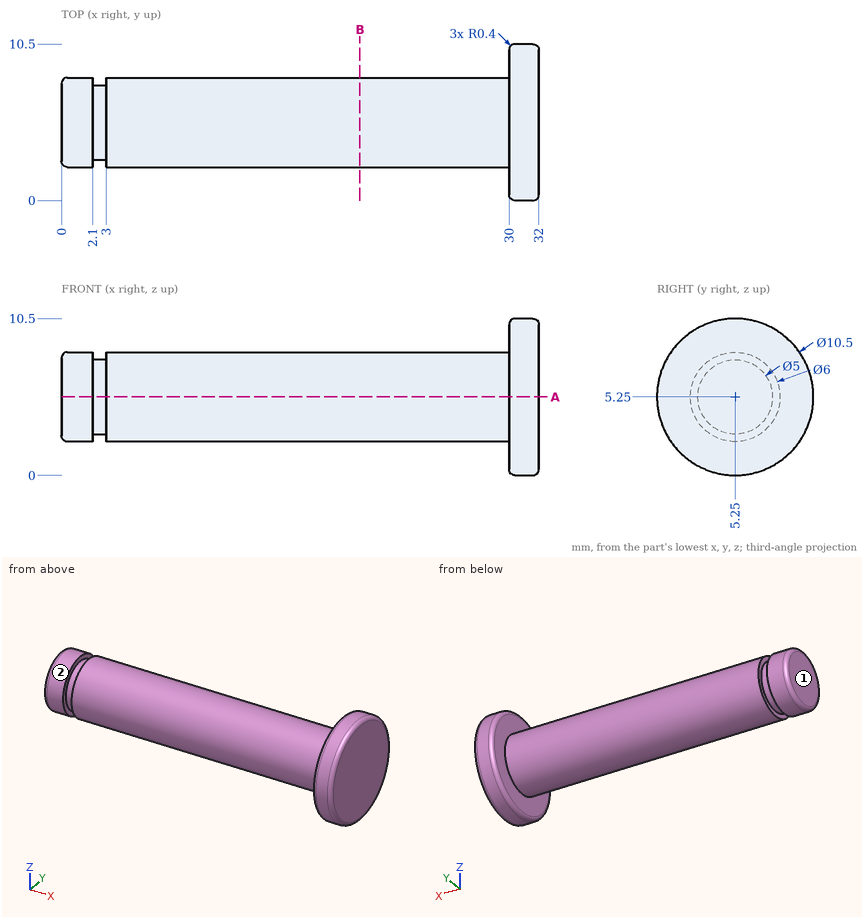
For this review, use the dimensioned drawing (mm, ordinates from the lowest corner) and the shaded views. A direction names the side the tool comes from. Coordinates: 2 decimals unless noted, no trailing zeros. Write each loop counter-clockwise with the first axis right and the second up, starting at its lowest first coordinate (ties: lowest second). Pieces come first, ordered by that corner, then holes. Notation, with made-up numbers: (67, 68.25) - (83, 68.25) arc R24 cw to (83, 103.25) - close; hole circle Ø1 at (40.25, 42.25). An arc over 180 degrees is marked (long way). Answer as a JSON object with one key per item and string values. Group by question number.
1. Clearance check with flat-ended pins moving along their axes: pin 1 Ø1 at (x, z) = (21.5, 4) entering from -Y; pin 2 Ø5 at (x, y) = (16.5, 7) entering from -Z; pin 3 Ø3 at (x, z) = (10, 1.5) entering from +Y. State where each tip first meets the part, or that it passes through.
2. Add section A-A (z = 5.25). Give the boundary of the cut face in (x, y).
3. Add section B-B (x = 20). Give the boundary of the cut face in (y, z).
4. Machinability: for the marked faces 1 and 2, which of the approach directions +Z, -Z, +X, -X, +Y, -Y give a long, thin tool a straight path to every point of the face, cutting with its end or side? Answer none if there is none.
5. To check wall thickness, follow probe 1 along X at (y, z) = (3.25, 7.75); probe 2 along Y at (x, z) = (23.5, 3.75). State the ranges of each line that lie inside material, in increasing order.
Findings:
{
 "1": {"pin 1": "y = 2.35", "pin 2": "z = 2.25", "pin 3": "y = 7.23"},
 "2": {"outline": "(0, 2.65) arc R0.4 ccw to (0.4, 2.25) - (2.1, 2.25) - (2.1, 2.75) - (3, 2.75) - (3, 2.25) - (30, 2.25) - (30, 0.4) arc R0.4 ccw to (30.4, 0) - (31.6, 0) arc R0.4 ccw to (32, 0.4) - (32, 10.1) arc R0.4 ccw to (31.6, 10.5) - (30.4, 10.5) arc R0.4 ccw to (30, 10.1) - (30, 8.25) - (3, 8.25) - (3, 7.75) - (2.1, 7.75) - (2.1, 8.25) - (0.4, 8.25) arc R0.4 ccw to (0, 7.85) - close"},
 "3": {"outline": "circle Ø6 at (5.25, 5.25)"},
 "4": {"face 1": "+Z, -Z, -X, +Y, -Y", "face 2": "-X"},
 "5": {"probe 1": "30 to 32", "probe 2": "2.65 to 7.85"}
}
